```python
from build123d import *

# Parameters (mm, degrees)
SKETCH2_W             = 60
SKETCH2_H             = 40
BOSS_EXTRUDE1_DEPTH   = 30
SHELL2_T              = -1.8
SKETCH2_6_W           = 22
SKETCH2_6_H           = 13
CUT_EXTRUDE4_DEPTH    = 30
F_6_0MM_DOWEL_HOLE1_D = 6.1


with BuildPart() as part:
    # Sketch2 → Boss-Extrude1 (new body)
    with BuildSketch(Plane(origin=(0, 0, 0), x_dir=(1, 0, 0), z_dir=(0, 1, 0))):
        with Locations((30, 20)):
            Rectangle(SKETCH2_W, SKETCH2_H)
    extrude(amount=BOSS_EXTRUDE1_DEPTH)

    # Shell2
    shell2_openings = [part.faces().sort_by_distance(p)[0] for p in [
        (30, 30, -20),
    ]]
    offset(amount=SHELL2_T, openings=shell2_openings, kind=Kind.INTERSECTION)

    # Sketch2<6> → Cut-Extrude4 (cut)
    with BuildSketch(Plane(origin=(0, 0, 0), x_dir=(1, 0, 0), z_dir=(0, 1, 0))):
        with Locations((30, 29.5)):
            Rectangle(SKETCH2_6_W, SKETCH2_6_H)
    extrude(amount=CUT_EXTRUDE4_DEPTH, mode=Mode.SUBTRACT)

    # Ø6.0mm Dowel Hole1 (through all)
    with Locations(Plane.ZY):
        with Locations((-29.5, 6.8)):
            Hole(F_6_0MM_DOWEL_HOLE1_D / 2)


solid = part.part
```
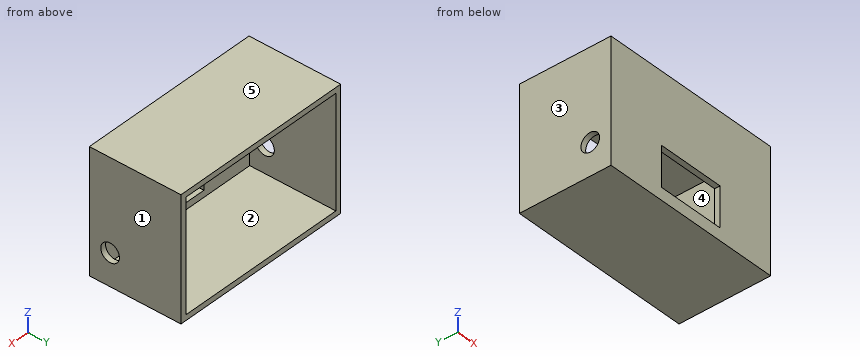
For this review, take the finished solid that the model builds, in its own axes (mm). Face numbers are marked on the shaded views. A direction names the side the tool comes from. Round coordinates to 2 decimals unless told otherwise and drop trailing zeros. Write each loop counter-clockwise with the first axis right and the second up, starting at its lowest first coordinate (ties: lowest second). Pieces come first, ordered by that corner, then holes. Notation, with made-up numbers: M 38.5,-2 L 49.5,-2 A27 ccw 49.5,14 Z; hole C -32.75,1 d2. An arc over 180 degrees is marked long. One line per item, written item: value. Start each with the question number.
(1) Machinability: for the marked faces 1 and 2, which of the approach directions +Z, -Z, +X, -X, +Y, -Y give a long, thin tool a straight path to every point of the face, cutting with its end or side? Answer none if there is none.
(2) We need section B-B (x = 39.5). Give the boundary of the cut face in (y, z).
(3) The part is to be moulded in two halves that separate along Z. For the marked faces 3, 4 and 5, say which applies: released by +Z, released by -Z, zero draft, split by the parting line, or undercut.
(4) Wall thickness on line 1 (X direction, y = 17.5, z = -29.5); line 2 (Y direction, x = 1, z = -29.5); line 3 (Z direction, x = 33, y = 13.5): over which ranges is each line inside the solid? List them lowest first.
(5) Insertion check: pin 1 (11 mm diameter, centred on x = 18, z = -15.5, fed in from +Y). The pin has a flat end and moves straight along its axis. Give the tip position at first contact, or say it passes through.
(6) We need section C-C (y = 6.8). Give the boundary of the cut face in (x, z).
(7) We need section A-A (z = -29.5). Give the boundary of the cut face in (x, y), and give its area (3 significant figures).
(8) We need section D-D (y = 21). Give the boundary of the cut face in (x, z).
Result:
1. face 1: +Z, -Z, +X, +Y, -Y
1. face 2: +Y
2. outline: M 0,-40 L 30,-40 L 30,-38.2 L 1.8,-38.2 L 1.8,-36 L 0,-36 Z; M 0,-23 L 1.8,-23 L 1.8,-1.8 L 30,-1.8 L 30,0 L 0,0 Z
3. face 3: zero draft
3. face 4: undercut
3. face 5: released by +Z
4. line 1: 0 to 1.8, 58.2 to 60
4. line 2: 0 to 3.75, 9.85 to 30
4. line 3: -40 to -38.2, -1.8 to 0
5. pin 1: y = 1.8
6. outline: M 0,-40 L 60,-40 L 60,-32.55 L 58.2,-32.55 L 58.2,-38.2 L 1.8,-38.2 L 1.8,-32.55 L 0,-32.55 Z; M 0,-26.45 L 1.8,-26.45 L 1.8,-1.8 L 58.2,-1.8 L 58.2,-26.45 L 60,-26.45 L 60,0 L 0,0 Z
7. outline: M 0,0 L 19,0 L 19,1.8 L 1.8,1.8 L 1.8,3.75 L 0,3.75 Z; M 0,9.85 L 1.8,9.85 L 1.8,30 L 0,30 Z; M 41,0 L 60,0 L 60,3.75 L 58.2,3.75 L 58.2,1.8 L 41,1.8 Z; M 58.2,9.85 L 60,9.85 L 60,30 L 58.2,30 Z
7. area: 148 mm²
8. outline: M 0,-40 L 60,-40 L 60,0 L 0,0 Z; hole M 1.8,-38.2 L 58.2,-38.2 L 58.2,-1.8 L 1.8,-1.8 Z
